```python
from build123d import *

# Parameters (mm, degrees)
ESQUISSE1_R             = 37
ESQUISSE1_R_2           = 1.5
ESQUISSE1_W             = 25
ESQUISSE1_H             = 3
BOSS_EXTRU_1_DEPTH      = 2
BOSS_EXTRU_2_DEPTH      = 15
ESQUISSE3_W             = 2
ESQUISSE3_H             = 28.4
BOSS_EXTRU_3_DEPTH      = 2.25
ESQUISSE5_W             = 2
ESQUISSE5_H             = 24.4
BOSS_EXTRU_4_DEPTH      = 2.25
ESQUISSE7_W             = 33.1
ESQUISSE7_H             = 28.4
BOSS_EXTRU_5_DEPTH      = 1
ESQUISSE8_W             = 15
ESQUISSE8_H             = 15
ENL_V_MAT_EXTRU_1_DEPTH = 3
ESQUISSE9_W             = 21
ESQUISSE9_H             = 2.5
ENL_V_MAT_EXTRU_2_DEPTH = 3
ESQUISSE10_R            = 1
ENL_V_MAT_EXTRU_3_DEPTH = 19
ENL_V_START             = -2
ESQUISSE11_R            = 37
ENL_V_MAT_EXTRU_4_DEPTH = 2


with BuildPart() as part:
    # Esquisse1 → Boss.-Extru.1 (new body)
    with BuildSketch(Plane.XY):
        Circle(ESQUISSE1_R)
        with Locations((0, 30)):
            Circle(ESQUISSE1_R_2, mode=Mode.SUBTRACT)
        with Locations((-22.874807889, 14.34375)):
            Circle(ESQUISSE1_R_2, mode=Mode.SUBTRACT)
        with Locations((-25.416453209, -15.9375)):
            Circle(ESQUISSE1_R_2, mode=Mode.SUBTRACT)
        with Locations((0, -27)):
            Circle(ESQUISSE1_R_2, mode=Mode.SUBTRACT)
        with Locations((25.416453209, -15.9375)):
            Circle(ESQUISSE1_R_2, mode=Mode.SUBTRACT)
        with Locations((22.874807889, 14.34375)):
            Circle(ESQUISSE1_R_2, mode=Mode.SUBTRACT)
        with Locations((0, -15.5)):
            Rectangle(ESQUISSE1_W, ESQUISSE1_H, mode=Mode.SUBTRACT)
    extrude(amount=BOSS_EXTRU_1_DEPTH)

    # Esquisse2 → Boss.-Extru.2 (add)
    with BuildSketch(Plane(origin=(0, 0, 0), x_dir=(-1, 0, 0), z_dir=(0, 0, -1))):
        Polygon((-16.75, 14.9), (-12.75, 14.9), (-12.75, -9.5), (12.35, -9.5), (12.35, 14.9), (16.35, 14.9), (16.35, -13.5), (-16.75, -13.5), align=None)
    extrude(amount=BOSS_EXTRU_2_DEPTH)

    # Esquisse3 → Boss.-Extru.3 (add)
    with BuildSketch(Plane(origin=(-12.35, 0, 0), x_dir=(0, 0, -1), z_dir=(1, 0, 0))):
        with Locations((9.625, 0.7)):
            Rectangle(ESQUISSE3_W, ESQUISSE3_H)
        with Locations((6.625, 0.7)):
            Rectangle(ESQUISSE3_W, ESQUISSE3_H)
    extrude(amount=BOSS_EXTRU_3_DEPTH)

    # Esquisse5 → Boss.-Extru.4 (add)
    with BuildSketch(Plane.ZY.offset(-12.75)):
        with Locations((-9.625, 2.7)):
            Rectangle(ESQUISSE5_W, ESQUISSE5_H)
        with Locations((-6.625, 2.7)):
            Rectangle(ESQUISSE5_W, ESQUISSE5_H)
    extrude(amount=BOSS_EXTRU_4_DEPTH)

    # Esquisse7 → Boss.-Extru.5 (add)
    with BuildSketch(Plane(origin=(0, 0, -15), x_dir=(-1, 0, 0), z_dir=(0, 0, -1))):
        with Locations((-0.2, 0.7)):
            Rectangle(ESQUISSE7_W, ESQUISSE7_H)
    extrude(amount=-BOSS_EXTRU_5_DEPTH)

    # Esquisse8 → Enlèv. mat.-Extru.1 (cut)
    with BuildSketch(Plane(origin=(0, 0, -15), x_dir=(-1, 0, 0), z_dir=(0, 0, -1))):
        Rectangle(ESQUISSE8_W, ESQUISSE8_H)
    extrude(amount=-ENL_V_MAT_EXTRU_1_DEPTH, mode=Mode.SUBTRACT)

    # Esquisse9 → Enlèv. mat.-Extru.2 (cut)
    with BuildSketch(Plane.XZ.offset(13.5)):
        with Locations((0, -5.65)):
            Rectangle(ESQUISSE9_W, ESQUISSE9_H)
    extrude(amount=-ENL_V_MAT_EXTRU_2_DEPTH, mode=Mode.SUBTRACT)

    # Esquisse10 → Enlèv. mat.-Extru.3 (cut)
    with BuildSketch(Plane.XY.offset(2)):
        with Locations((-14.35, 8.9)):
            Circle(ESQUISSE10_R)
        with Locations((-14.35, -11.5)):
            Circle(ESQUISSE10_R)
        with Locations((14.75, -11.5)):
            Circle(ESQUISSE10_R)
        with Locations((14.75, 8.9)):
            Circle(ESQUISSE10_R)
    extrude(amount=-ENL_V_MAT_EXTRU_3_DEPTH, mode=Mode.SUBTRACT)

    # Esquisse11 → Enlèv. mat.-Extru.4 (cut)
    with BuildSketch(Plane.XY.offset(2).offset(ENL_V_START)):
        Circle(ESQUISSE11_R)
    extrude(amount=ENL_V_MAT_EXTRU_4_DEPTH, mode=Mode.SUBTRACT)


solid = part.part
```
The model under review builds one solid part; all positions refer to its coordinate system, in mm. A direction names the side the tool comes from. Round coordinates to 2 decimals unless told otherwise and drop trailing zeros. Write each loop counter-clockwise with the first axis right and the second up, starting at its lowest first coordinate (ties: lowest second). Pieces come first, ordered by that corner, then holes.
(1) Machinability: for faces 1 (the flat face through (12, 3, -5.625)), 2 (the flat face through (0.1, 7.5, -14.5)), 3 (the flat face through (0, -12, -6.9)), 4 (the flat face through (12, 3, -10.625)), 5 (the flat face through (-16.35, 1, -7)), which of the approach directions +Z, -Z, +X, -X, +Y, -Y give a long, thin tool a straight path to every point of the face, cutting with its end or side? Answer none if there is none.
(2) We need section A-A on y = -11.5. Give the boundary of the cut face in (x, z).
(3) We need section D-D on y = -4.5. Give the boundary of the cut face in (x, z) (3 decimals), and give its area (3 significant figures).
(4) We need section B-B on x = 4. Give the boundary of the cut face in (y, z), and give its area (3 significant figures).
(5) Mouldability with a two-part tool opening along Y and no side actions: class faces 6 (the cylindrical face through (15.704, -11.2, -7.395)), 7 (the flat face through (11, 14.9, -9)), 8 (the flat face through (0, -11, 0)), 9 (the flat face through (7.5, -0.1, -14.5)) as +Y half, -Y half, draft (parallel to the pull), parting line (faces both ways), or undercut.
(6) Insertion check: pin 1 (4 mm diameter, centred on x = 4, z = -11, fed in from +Y). The pin has a flat end and moves straight along its axis. Give the tip position at first contact, or say it passes through.
(7) We need section C-C on z = -9.5. Give the boundary of the cut face in (x, y), and give its area (3 significant figures).
(8) Wall thickness on L1, parallel to Z at x = -11.5, y = 5.5 (3 decimals); L2, parallel to X at y = -3.75, z = -7; L3, parallel to X at y = 0, z = -13.25: over which ranges is each line inside the solid? List them lowest first.
Findings below:
1. face 1: +Z, +Y
1. face 2: +Z, -Z
1. face 3: -Y
1. face 4: +Y
1. face 5: +Z, -Z, -X, +Y, -Y
2. outline: (-16.35, -15) - (-15.35, -15) - (-15.35, 0) - (-16.35, 0) - close; (-13.35, -15) - (13.75, -15) - (13.75, 0) - (-13.35, 0) - close; (15.75, -15) - (16.75, -15) - (16.75, 0) - (15.75, 0) - close; hole (-10.5, -6.9) - (10.5, -6.9) - (10.5, -4.4) - (-10.5, -4.4) - close
3. outline: (-16.35, -15) - (-7.5, -15) - (-7.5, -14) - (-12.35, -14) - (-12.35, -10.625) - (-10.1, -10.625) - (-10.1, -8.625) - (-12.35, -8.625) - (-12.35, -7.625) - (-10.1, -7.625) - (-10.1, -5.625) - (-12.35, -5.625) - (-12.35, 0) - (-16.35, 0) - close; (7.5, -15) - (16.75, -15) - (16.75, 0) - (12.75, 0) - (12.75, -5.625) - (10.5, -5.625) - (10.5, -7.625) - (12.75, -7.625) - (12.75, -8.625) - (10.5, -8.625) - (10.5, -10.625) - (12.75, -10.625) - (12.75, -14) - (7.5, -14) - close
3. area: 148 mm2
4. outline: (-13.5, -15) - (-7.5, -15) - (-7.5, -14) - (-9.5, -14) - (-9.5, 0) - (-13.5, 0) - (-13.5, -4.4) - (-10.5, -4.4) - (-10.5, -6.9) - (-13.5, -6.9) - close; (7.5, -15) - (14.9, -15) - (14.9, -14) - (7.5, -14) - close
4. area: 61.9 mm2
5. face 6: undercut
5. face 7: +Y half
5. face 8: draft
5. face 9: undercut
6. pin 1: stops at y = -9.5
7. outline: (-16.35, -13.5) - (16.75, -13.5) - (16.75, 14.9) - (10.5, 14.9) - (10.5, -9.5) - (-10.1, -9.5) - (-10.1, 14.9) - (-16.35, 14.9) - close; hole circle Ø2 at (-14.35, -11.5); hole circle Ø2 at (-14.35, 8.9); hole circle Ø2 at (14.75, -11.5); hole circle Ø2 at (14.75, 8.9)
7. area: 425 mm2
8. L1: z = -15 to -14, -10.625 to -8.625, -7.625 to -5.625
8. L2: x = -16.35 to -10.1, 10.5 to 16.75
8. L3: x = -16.35 to -12.35, 12.75 to 16.75
